from build123d import *

# Parameters (mm, degrees)
SKETCH1_W           = 86
SKETCH1_H           = 86
BOSS_EXTRUDE1_DEPTH = 23
SHELL1_T            = -3
SKETCH2_W           = 9
SKETCH2_H           = 20
CUT_EXTRUDE1_DEPTH  = 3


with BuildPart() as part:
    # Sketch1 → Boss-Extrude1 (new body)
    with BuildSketch(Plane(origin=(0, 0, 0), x_dir=(1, 0, 0), z_dir=(0, 1, 0))):
        with Locations((-6.49444668, 4.080083427)):
            Rectangle(SKETCH1_W, SKETCH1_H)
    extrude(amount=BOSS_EXTRUDE1_DEPTH)

    # Shell1
    shell1_openings = [part.faces().sort_by_distance(p)[0] for p in [
        (-6.49444668, 23, -4.080083427),
        (-6.49444668, 11.5, -47.080083427),
    ]]
    offset(amount=SHELL1_T, openings=shell1_openings, kind=Kind.INTERSECTION)

    # Sketch2 → Cut-Extrude1 (cut)
    with BuildSketch(Plane.ZY.offset(49.49444668)):
        with Locations((-7.580083427, 13)):
            Rectangle(SKETCH2_W, SKETCH2_H)
    extrude(amount=-CUT_EXTRUDE1_DEPTH, mode=Mode.SUBTRACT)


solid = part.part
The listing builds one solid part. Answer for the finished solid, in the listing's coordinates (mm). A direction names the side the tool comes from. Round coordinates to 2 decimals unless told otherwise and drop trailing zeros. Write each loop counter-clockwise with the first axis right and the second up, starting at its lowest first coordinate (ties: lowest second). Pieces come first, ordered by that corner, then holes. Notation, with made-up numbers: (8.25, 79.25) - (40.25, 79.25) arc R20 cw to (40.25, 114.25) - close; hole circle Ø7 at (-26, 80). An arc over 180 degrees is marked (long way). Use one line per item in the form item = value. Start each with the question number.
Item 1: Determine the mould class of faces 1 (the flat face through (-46.494, 13, 17)), 2 (the flat face through (36.506, 11, -3)), 3 (the flat face through (-7, 0, -5)) for opening direction X: +X half, -X half, draft (parallel to the pull), parting line (faces both ways), or undercut.
Item 2: A cutting plane is placed at B-B (y = 15.75). Write down the section's boundary in (x, z).
Item 3: A cutting plane is placed at C-C (x = -29). Write down the section's boundary in (y, z), plus the area to 3 significant figures.
Item 4: A cutting plane is placed at D-D (z = -8). Write down the section's boundary in (x, y), plus the area to 3 significant figures.
Item 5: Flat-ended cylindrical pins translate along their axes: pin 1 Ø1 at (x, y) = (-23, 4) entering from -Z; pin 2 Ø1.5 at (x, z) = (-39, -11.5) entering from -Y. Find the tip coordinate at first contact, or state that the pin passes through.
Item 6: A cutting plane is placed at A-A (z = 2). Write down the section's boundary in (x, y).
Item 7: Find the intervals of material crossed by line 1 (X direction, y = 10, z = 8.5); line 2 (Z direction, x = -13.5, y = 5.25); line 3 (Y direction, x = 10, z = -29), in increasing order. Write a range as [from, to].
Item 8: A tool of negligible diameter and unlimited length cuts with its end or side. For faces 4 (the flat face through (-7, 13, 35.92)), 5 (the flat face through (-48, 13, -3.08)), 6 (the flat face through (-7, 1, -47.08)), from which of +Z, -Z, +X, -X, +Y, -Y can it reach the whole face along a straight path? Write none if from no direction.
The answers:
q1.face_1 = undercut
q1.face_2 = +X half
q1.face_3 = draft
q2.outline = (-49.49, -47.08) - (-46.49, -47.08) - (-46.49, -12.08) - (-49.49, -12.08) - close; (-49.49, -3.08) - (-46.49, -3.08) - (-46.49, 35.92) - (33.51, 35.92) - (33.51, -47.08) - (36.51, -47.08) - (36.51, 38.92) - (-49.49, 38.92) - close
q3.outline = (0, -47.08) - (3, -47.08) - (3, 35.92) - (23, 35.92) - (23, 38.92) - (0, 38.92) - close
q3.area = 318 mm^2
q4.outline = (-49.49, 0) - (36.51, 0) - (36.51, 23) - (33.51, 23) - (33.51, 3) - (-49.49, 3) - close
q4.area = 318 mm^2
q5.pin_1 = 35.92
q5.pin_2 = 0
q6.outline = (-49.49, 0) - (36.51, 0) - (36.51, 23) - (33.51, 23) - (33.51, 3) - (-46.49, 3) - (-46.49, 23) - (-49.49, 23) - close
q7.line_1 = [-49.49, -46.49], [33.51, 36.51]
q7.line_2 = [35.92, 38.92]
q7.line_3 = [0, 3]
q8.face_4 = -Z, +Y
q8.face_5 = -X, +Y
q8.face_6 = -Z, +X, -X, +Y, -Y
